```python
from build123d import *

# Parameters (mm, degrees)
F1_DEPTH    = 20
F3_DEPTH    = 70
F4_R        = 1.5
F5_DEPTH    = 6
F6_T1_DEPTH = 20
F6_T3_DEPTH = 20
F6_T5_DEPTH = 15.2864150343
F6_T7_DEPTH = 15.2864150343
F6_T9_DEPTH = 35
F8_DEPTH    = 25
F9_DEPTH    = 25


# Not quite as in the source:
# - a fillet or chamfer that OpenCascade refuses, or shapes differently, is made with other operations: its cross-section is extruded or revolved along the edge and cut away or added


with BuildPart() as f1:
    # F0 (on Right) → F1 (new body)
    with BuildSketch(Plane.YZ):
        Polygon((0, -26.8219177697), (0, 23.6780822303), (16, 23.6780822303), (16, 28.6780822303), (-6, 28.6780822303), (-6, -31.8219177697), (16, -31.8219177697), (16, -26.8219177697), align=None)
    extrude(amount=F1_DEPTH)

    # F2 (on face) → F3 (cut)
    with BuildSketch(Plane.XY.offset(28.6780822303)):
        with BuildLine():
            ThreePointArc((4.5, 13.4109126902), (6.7375618827, 6.9418292298), (12.25, 11))
            ThreePointArc((12.25, 11), (12.0581707702, 12.2624381173), (11.5, 13.4109126902))
            ThreePointArc((11.5, 13.4109126902), (8, 15.25), (4.5, 13.4109126902))
        make_face()
        with BuildLine():
            ThreePointArc((4.5, 13.4109126902), (8, 15.25), (11.5, 13.4109126902))
            Line((11.5, 13.4109126902), (12.5, 16))
            Line((12.5, 16), (3.5, 16))
            Line((3.5, 16), (4.5, 13.4109126902))
        make_face()
    extrude(amount=-F3_DEPTH, mode=Mode.SUBTRACT)

    # F4 (on face) → F5 (join)
    with BuildSketch(Plane.XZ.offset(6)):
        Polygon((20, 16.1780822303), (20, -6.8219177697), (30, -6.8219177697), (47, -6.8219177697), (47, 16.1780822303), (30, 16.1780822303), align=None)
        with Locations((31.5, 4.6780822303)):
            Circle(F4_R, mode=Mode.SUBTRACT)
        with Locations((41.5, 4.6780822303)):
            Circle(F4_R, mode=Mode.SUBTRACT)
        Polygon((30, -6.8219177697), (20, -6.8219177697), (20, -31.8219177697), align=None)
        Polygon((20, 28.1780822303), (20, 16.1780822303), (30, 16.1780822303), align=None)
    extrude(amount=-F5_DEPTH)

    # F6: fillet of radius 3 on 10 edges, made by hand

    # F6_s2 → F6_t1 (cut)
    with BuildSketch(Plane.XY.offset(16.1780822303)):
        with BuildLine():
            ThreePointArc((17, 16), (19.1213203436, 15.1213203436), (20, 13))
            Line((20, 13), (20, 16))
            Line((20, 16), (17, 16))
        make_face()
        with BuildLine():
            ThreePointArc((0, 13), (0.8786796564, 15.1213203436), (3, 16))
            Line((3, 16), (0, 16))
            Line((0, 16), (0, 13))
        make_face()
    extrude(amount=F6_T1_DEPTH, mode=Mode.SUBTRACT)

    # F6_s4 → F6_t3 (cut)
    with BuildSketch(Plane.XY.offset(-39.3219177697)):
        with BuildLine():
            ThreePointArc((20, 13), (19.1213203436, 15.1213203436), (17, 16))
            Line((17, 16), (20, 16))
            Line((20, 16), (20, 13))
        make_face()
        with BuildLine():
            ThreePointArc((0, 13), (0.8786796564, 15.1213203436), (3, 16))
            Line((3, 16), (0, 16))
            Line((0, 16), (0, 13))
        make_face()
    extrude(amount=F6_T3_DEPTH, mode=Mode.SUBTRACT)

    # F6_s6 → F6_t5 (cut)
    with BuildSketch(Plane.XY.offset(18.5348747132)):
        with BuildLine():
            ThreePointArc((11.7587690029, 14.0808882317), (12.8606193241, 15.4741326455), (14.5572830069, 16))
            Line((14.5572830069, 16), (12.5, 16))
            Line((12.5, 16), (11.7587690029, 14.0808882317))
        make_face()
        with BuildLine():
            ThreePointArc((1.4427169931, 16), (3.1393806759, 15.4741326455), (4.2412309971, 14.0808882317))
            Line((4.2412309971, 14.0808882317), (3.5, 16))
            Line((3.5, 16), (1.4427169931, 16))
        make_face()
    extrude(amount=F6_T5_DEPTH, mode=Mode.SUBTRACT)

    # F6_s8 → F6_t7 (cut)
    with BuildSketch(Plane.XY.offset(-36.9651252868)):
        with BuildLine():
            ThreePointArc((14.5572830069, 16), (12.8606193241, 15.4741326455), (11.7587690029, 14.0808882317))
            Line((11.7587690029, 14.0808882317), (12.5, 16))
            Line((12.5, 16), (14.5572830069, 16))
        make_face()
        with BuildLine():
            ThreePointArc((4.2412309971, 14.0808882317), (3.1393806759, 15.4741326455), (1.4427169931, 16))
            Line((1.4427169931, 16), (3.5, 16))
            Line((3.5, 16), (4.2412309971, 14.0808882317))
        make_face()
    extrude(amount=F6_T7_DEPTH, mode=Mode.SUBTRACT)

    # F6_s10 → F6_t9 (cut)
    with BuildSketch(Plane.YZ.offset(-7.5)):
        with BuildLine():
            ThreePointArc((-3, 28.6780822303), (-5.1213203436, 27.7994025739), (-6, 25.6780822303))
            Line((-6, 25.6780822303), (-6, 28.6780822303))
            Line((-6, 28.6780822303), (-3, 28.6780822303))
        make_face()
        with BuildLine():
            ThreePointArc((-6, -28.8219177697), (-5.1213203436, -30.9432381132), (-3, -31.8219177697))
            Line((-3, -31.8219177697), (-6, -31.8219177697))
            Line((-6, -31.8219177697), (-6, -28.8219177697))
        make_face()
    extrude(amount=F6_T9_DEPTH, mode=Mode.SUBTRACT)

    # F7 (on face) → F8 (cut)
    with BuildSketch(Plane.XZ.offset(6)):
        Polygon((0, 6.1780822303), (0, -23.8219177697), (8, -18.8219177697), (8, 1.1780822303), align=None)
    extrude(amount=-F8_DEPTH, mode=Mode.SUBTRACT)

    # F7 (on face) → F9 (cut)
    with BuildSketch(Plane.XZ.offset(6)):
        Polygon((0, 6.1780822303), (0, -23.8219177697), (8, -18.8219177697), (8, 1.1780822303), align=None)
    extrude(amount=-F9_DEPTH, mode=Mode.SUBTRACT)


solid = f1.part
```
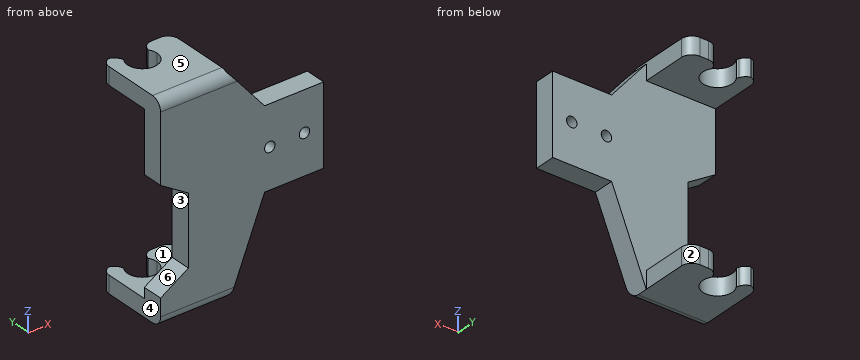
Could you check a few things on this model? Use its own coordinates, in mm. Face numbers are marked on the shaded views. A direction names the side the tool comes from. Coordinates: 2 decimals unless noted, no trailing zeros. Loops run counter-clockwise (first coordinate to the right, second up) from the corner with the lowest first, then second, coordinate; pieces in that order, holes last.
1) Which directions (+Z, -Z, +X, -X, +Y, -Y) give clear straight access to the entire face, cutting with the end or side of a thin tool? Please do the marked faces 1, 2 and 3.
Reported:
face 1: +X, -X, +Y
face 2: +Z, -Z, +X, +Y
face 3: -X, +Y, -Y
2) Imagine slicing it at B-B (x = 31.5). List the corners of the cut face in (y, z) for me.
Reported:
outline: (-6, -6.82) - (0, -6.82) - (0, 3.18) - (-6, 3.18) - close; (-6, 6.18) - (0, 6.18) - (0, 16.18) - (-6, 16.18) - close
3) Thinking about a two-plate mould opening in Z: for the marked faces 4, 5 and 6, which applies, released by +Z, released by -Z, zero draft, split by the parting line, or undercut?
Reported:
face 4: zero draft
face 5: released by +Z
face 6: undercut
4) Imagine slicing it at A-A (y = 5.25). List the corners of the cut face in (x, z) for me, and give its area (3 significant figures).
Reported:
outline: (0, -31.82) - (20, -31.82) - (20, -26.82) - (0, -26.82) - close; (0, 23.68) - (20, 23.68) - (20, 28.68) - (0, 28.68) - close
area: 200 mm2
5) Will these pins go through, and if not, where does the flat tip stop? pin 1 Ø4 at (y, z) = (4.5, 26.5) entering from +X; pin 2 Ø6 at (x, z) = (24.5, -12) entering from +Y; pin 3 Ø6.5 at (x, y) = (36, -3.5) entering from -Z; pin 4 Ø5 at (x, y) = (39, 3) entering from +Z.
Reported:
pin 1: stops at x = 20
pin 2: stops at y = 0
pin 3: stops at z = -6.82
pin 4: passes through
6) Imagine slicing it at C-C (z = 9). List the corners of the cut face in (x, y) for me.
Reported:
outline: (0, -6) - (47, -6) - (47, 0) - (0, 0) - close
7) Please list where these lines run through material, in increasing order: line 1 along Z through (x, y) = (41.5, -1.9); line 2 along X through (y, z) = (11, 26.85); line 3 along X through (y, z) = (3, 25).
Reported:
line 1: z = -6.82 to 3.18, 6.18 to 16.18
line 2: x = 0 to 3.75, 12.25 to 20
line 3: x = 0 to 20
8) Imagine slicing it at D-D (x = 19). List the corners of the cut face in (y, z) for me, and give its area (3 significant figures).
Reported:
outline: (-6, -28.82) arc R3 ccw to (-3, -31.82) - (15.24, -31.82) - (15.24, -26.82) - (0, -26.82) - (0, 23.68) - (15.24, 23.68) - (15.24, 28.68) - (-3, 28.68) arc R3 ccw to (-6, 25.68) - close
area: 511 mm2
